Autodesk Inventor part; units mm, degrees
ref_plane "YZ Plane" through (0, 0, 0) normal (1, 0, 0) x (0, 1, 0)
ref_plane "XZ Plane" through (0, 0, 0) normal (0, 1, 0) x (-1, 0, 0)
ref_plane "XY Plane" through (0, 0, 0) normal (0, 0, 1) x (1, 0, 0)
sketch "スケッチ1" plane through (0, 0, 0) normal (0, 1, 0) x (-1, 0, 0)
  line L0 (10.75, 21.6) -> (-10.75, 21.6)
  line L1 (-10.75, 21.6) -> (-10.75, -21.6)
  line L2 (-10.75, -21.6) -> (10.75, -21.6)
  line L3 (10.75, -21.6) -> (10.75, 21.6)
  line L4 (0, -30.24) -> (0, 30.24)
  line L5 (-15.05, 0) -> (15.05, 0)
  point P0 (0, 0)
  dimension "d0" = 21.5
  dimension "d1" = 43.2
extrude "押し出し1" add sketch "スケッチ1" along normal blind 16
sketch "スケッチ2" plane through (0, 16, 0) normal (0, 1, 0) x (1, 0, 0)
  line L0 (-10.75, -28.6) -> (10.75, -28.6)
  line L1 (10.75, -28.6) -> (10.75, 28.6)
  line L2 (10.75, 28.6) -> (-10.75, 28.6)
  line L3 (-10.75, 28.6) -> (-10.75, -28.6)
  line L4 (15.155, 0) -> (-15.155, 0)
  point P0 (0, 0)
  point P1 (-10.75, -21.6)
  point P2 (10.75, -21.6)
  dimension "d4" = 57.2
extrude "押し出し2" add sketch "スケッチ2" along normal blind 5
sketch "スケッチ3" plane through (0, 21, 0) normal (0, 1, 0) x (1, 0, 0)
  circle A0 centre (-6, -25.6) radius 1.5
  circle A1 centre (6, -25.6) radius 1.5
  circle A2 centre (-6, 25.6) radius 1.5
  circle A3 centre (6, 25.6) radius 1.5
  line L0 (15.05, 0) -> (-15.05, 0)
  line L1 (0, 40.04) -> (0, -40.04)
  point P0 (0, 0)
  dimension "d9" = 3
  dimension "d10" = 3
  dimension "d11" = 3
  dimension "d12" = 3
  dimension "d13" = 12
  dimension "d14" = 12
  dimension "d15" = 51.2
  dimension "d16" = 51.2
extrude "押し出し3" cut sketch "スケッチ3" against normal up to next
sketch "スケッチ4" plane through (0, 21, 0) normal (0, 1, 0) x (1, 0, 0)
  line L0 (10.75, 21.6) -> (-10.75, 21.6)
  line L1 (-10.75, -21.6) -> (10.75, -21.6)
  line L2 (-10.75, 28.6) -> (-10.75, -28.6)
  line L3 (10.75, -28.6) -> (10.75, 28.6)
  point P0 (0, 0)
extrude "押し出し4" add sketch "スケッチ4" along normal blind 2
sketch "スケッチ5" plane through (0, 23, 0) normal (0, 1, 0) x (1, 0, 0)
  circle A0 centre (0, -11.4) radius 3
  circle A1 centre (6, -25.6) radius 1.5
  line L0 (0, 40.04) -> (0, -40.04)
  point P0 (0, 0)
  dimension "d21" = 14.2
  dimension "d22" = 6
extrude "押し出し5" add sketch "スケッチ5" along normal blind 3.6 contours A0 L0 | L0 A0
properties part number "servo"
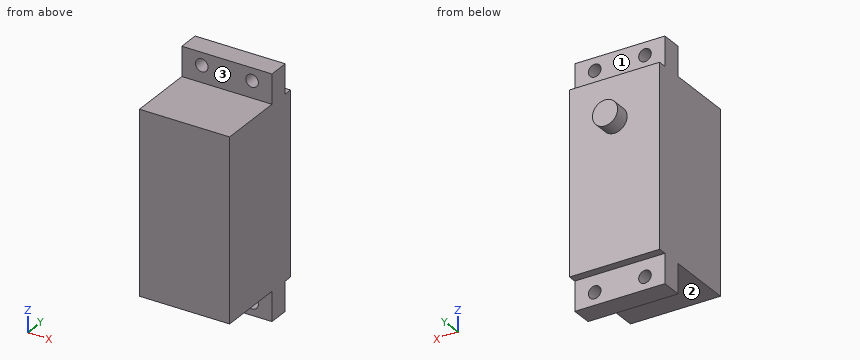
Part model, mm, in its own coordinate system. Face numbers are marked on the shaded views. A direction names the side the tool comes from. Coordinates: 2 decimals unless noted, no trailing zeros. Order: outer loops, then holes, each group sorted by start corner. A loop starts at its lowest first (then second) coordinate and runs counter-clockwise, first axis right, second up. Notation, with made-up numbers: (63.25, -37.5) - (76.25, -37.5) arc R26 ccw to (76.25, -10.5) - close; hole circle Ø1 at (0, -6). An arc over 180 degrees is marked (long way). Return JSON: item names as keys, results as strings. Group by question number.
Item 1: Cut at B-B (x = 6). List the corners of the cut face in (y, z), plus the area to 3 significant figures.
Item 2: Pin check, flat tips, straight feed: pin 1 (2 mm diameter, centred on x = 0.5, z = -24.5, fed in from -Y); pin 2 (5 mm diameter, centred on x = 3, z = -12.5, fed in from -Y); pin 3 (5.5 mm diameter, centred on x = -2, z = -24.5, fed in from +Y); pin 4 (2 mm diameter, centred on x = -3.5, y = 9.5, fed in from -Z). Stop position of each tip, or through.
Item 3: Drill centre lines: probe 1 along X at (y, z) = (18.25, -25.6); probe 2 along Y at (x, z) = (0.25, 21.5); probe 3 along Z at (x, y) = (-7.5, 8). Where is each one in solid material? Low to high. Write a range as from..to.
Item 4: Cut at C-C (x = 0). List the corners of the cut face in (y, z), plus the area to 3 significant figures.
Item 5: Cut at A-A (z = -25.6). List the corners of the cut face in (x, y).
Item 6: Cut at D-D (z = 11.4). List the corners of the cut face in (x, y), plus the area to 3 significant figures.
Item 7: Which spindle directions (+Z, -Z, +X, -X, +Y, -Y) get a long thin tool onto all of the face, cutting with end or side? Do the marked faces 1, 2 and 3. Say none if no direction does.
Check values:
{
 "1": {"outline": "(0, -21.6) - (16, -21.6) - (16, -24.1) - (21, -24.1) - (21, -21.6) - (23, -21.6) - (23, 21.6) - (21, 21.6) - (21, 24.1) - (16, 24.1) - (16, 21.6) - (0, 21.6) - close; (16, -28.6) - (21, -28.6) - (21, -27.1) - (16, -27.1) - close; (16, 27.1) - (21, 27.1) - (21, 28.6) - (16, 28.6) - close", "area": "1,030 mm2"},
 "2": {"pin 1": "stops at y = 16", "pin 2": "stops at y = 0", "pin 3": "stops at y = 21", "pin 4": "stops at z = -21.6"},
 "3": {"probe 1": "x = -10.75..-7.5, -4.5..4.5, 7.5..10.75", "probe 2": "y = 0..23", "probe 3": "z = -21.6..21.6"},
 "4": {"outline": "(0, -21.6) - (16, -21.6) - (16, -28.6) - (21, -28.6) - (21, -21.6) - (23, -21.6) - (23, 8.4) - (26.6, 8.4) - (26.6, 14.4) - (23, 14.4) - (23, 21.6) - (21, 21.6) - (21, 28.6) - (16, 28.6) - (16, 21.6) - (0, 21.6) - close", "area": "1,090 mm2"},
 "5": {"outline": "(-10.75, 16) - (-7.5, 16) - (-7.5, 21) - (-10.75, 21) - close; (-4.5, 16) - (4.5, 16) - (4.5, 21) - (-4.5, 21) - close; (7.5, 16) - (10.75, 16) - (10.75, 21) - (7.5, 21) - close"},
 "6": {"outline": "(-10.75, 0) - (10.75, 0) - (10.75, 23) - (3, 23) - (3, 26.6) - (-3, 26.6) - (-3, 23) - (-10.75, 23) - close", "area": "516 mm2"},
 "7": {"face 1": "+Z, +X, -X, +Y", "face 2": "-Z, +X, -X, -Y", "face 3": "+Z, +X, -X, -Y"}
}
